Verification items for the finished model (mm, model axes). Face numbers are marked on the shaded views. A direction names the side the tool comes from. Coordinates: 2 decimals unless noted, no trailing zeros. Write each loop counter-clockwise with the first axis right and the second up, starting at its lowest first coordinate (ties: lowest second). Pieces come first, ordered by that corner, then holes. Notation, with made-up numbers: M 84,82 L 116,82 A20 cw 116,103 Z; hole C 82,36 d1. An arc over 180 degrees is marked long. One line per item, written item: value.
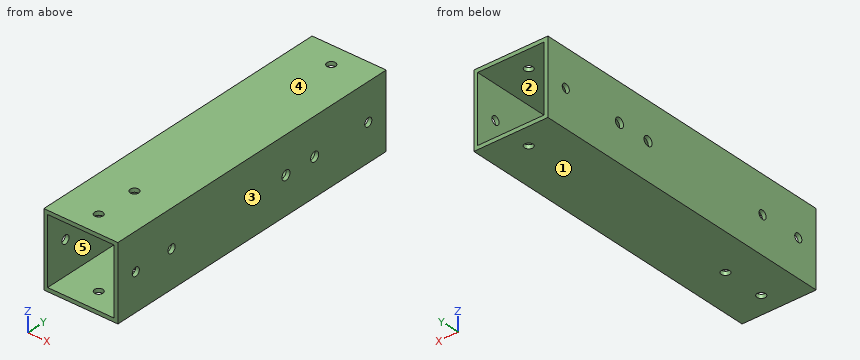
```python
from build123d import *

# Parameters (mm, degrees)
SKETCH1_W           = 35
SKETCH1_H           = 35
SKETCH1_W_2         = 31.4
SKETCH1_H_2         = 31.4
BOSS_EXTRUDE1_DEPTH = 150
SKETCH3_R           = 2
CUT_EXTRUDE1_DEPTH  = 156.020159979
SKETCH4_R           = 2
CUT_EXTRUDE2_DEPTH  = 156.020159979
SKETCH7_R           = 2
CUT_EXTRUDE5_DEPTH  = 40
SKETCH9_R           = 2
CUT_EXTRUDE6_DEPTH  = 40
SKETCH11_R          = 2.25
CUT_EXTRUDE8_DEPTH  = 156.020159979


with BuildPart() as part:
    # Sketch1 → Boss-Extrude1 (new body)
    with BuildSketch(Plane(origin=(0, 0, 0), x_dir=(1, 0, 0), z_dir=(0, 1, 0))):
        Rectangle(SKETCH1_W, SKETCH1_H)
        Rectangle(SKETCH1_W_2, SKETCH1_H_2, mode=Mode.SUBTRACT)
    extrude(amount=BOSS_EXTRUDE1_DEPTH)

    # Sketch3 → Cut-Extrude1 (cut, through all)
    with BuildSketch(Plane.XY.offset(17.5)):
        with Locations((0, 10)):
            Circle(SKETCH3_R)
        with Locations((0, 30)):
            Circle(SKETCH3_R)
    extrude(amount=-CUT_EXTRUDE1_DEPTH, mode=Mode.SUBTRACT)

    # Sketch4 → Cut-Extrude2 (cut, through all)
    with BuildSketch(Plane(origin=(17.5, 0, 0), x_dir=(0, 0, -1), z_dir=(1, 0, 0))):
        with Locations((0, 10)):
            Circle(SKETCH4_R)
        with Locations((0, 30)):
            Circle(SKETCH4_R)
    extrude(amount=-CUT_EXTRUDE2_DEPTH, mode=Mode.SUBTRACT)

    # Sketch7 → Cut-Extrude5 (cut)
    with BuildSketch(Plane(origin=(17.5, 0, 0), x_dir=(0, 0, -1), z_dir=(1, 0, 0))):
        with Locations((0, 140)):
            Circle(SKETCH7_R)
    extrude(amount=-CUT_EXTRUDE5_DEPTH, mode=Mode.SUBTRACT)

    # Sketch9 → Cut-Extrude6 (cut)
    with BuildSketch(Plane.XY.offset(17.5)):
        with Locations((0, 140)):
            Circle(SKETCH9_R)
    extrude(amount=-CUT_EXTRUDE6_DEPTH, mode=Mode.SUBTRACT)

    # Sketch11 → Cut-Extrude8 (cut, through all)
    with BuildSketch(Plane(origin=(17.5, 0, 0), x_dir=(0, 0, -1), z_dir=(1, 0, 0))):
        with Locations((0, 110)):
            Circle(SKETCH11_R)
        with Locations((0, 94)):
            Circle(SKETCH11_R)
    extrude(amount=-CUT_EXTRUDE8_DEPTH, mode=Mode.SUBTRACT)


solid = part.part
```
Item 1: Draft check along X on the marked faces 1, 2 and 3. Enter one of: released by +X, released by -X, zero draft, split by the parting line, or undercut.
The answers:
face 1: zero draft
face 2: undercut
face 3: released by +X
Item 2: Cross-section at D-D, the plane x = 0. Give the number of separate pieces and of enclosed holes in the cut face, and give its area (3 significant figures).
The answers:
separate pieces: 8
enclosed holes: 0
area: 497 mm²
Item 3: Cross-section at A-A, the plane y = 30. Enter the section's corners in (x, z).
The answers:
outline: M -17.5,-17.5 L -2,-17.5 L -2,-15.7 L -15.7,-15.7 L -15.7,-2 L -17.5,-2 Z; M -17.5,2 L -15.7,2 L -15.7,15.7 L -2,15.7 L -2,17.5 L -17.5,17.5 Z; M 2,-17.5 L 17.5,-17.5 L 17.5,-2 L 15.7,-2 L 15.7,-15.7 L 2,-15.7 Z; M 2,15.7 L 15.7,15.7 L 15.7,2 L 17.5,2 L 17.5,17.5 L 2,17.5 Z
Item 4: Cross-section at C-C, the plane y = 110. Enter the section's corners in (x, z).
The answers:
outline: M -17.5,-17.5 L 17.5,-17.5 L 17.5,-2.25 L 15.7,-2.25 L 15.7,-15.7 L -15.7,-15.7 L -15.7,-2.25 L -17.5,-2.25 Z; M -17.5,2.25 L -15.7,2.25 L -15.7,15.7 L 15.7,15.7 L 15.7,2.25 L 17.5,2.25 L 17.5,17.5 L -17.5,17.5 Z
Item 5: Scan lines: line 1 (Y direction, x = -16, z = 0); line 2 (Y direction, x = 0, z = -16.35); line 3 (X direction, y = 137, z = -0.5). Record each from-to range of solid material in increasing order.
The answers:
line 1: y = 0 to 8, 12 to 28, 32 to 91.75, 96.25 to 107.75, 112.25 to 138, 142 to 150
line 2: y = 0 to 8, 12 to 28, 32 to 138, 142 to 150
line 3: x = -17.5 to -15.7, 15.7 to 17.5
Item 6: Cross-section at B-B, the plane z = 14. Enter the section's corners in (x, y).
The answers:
outline: M -17.5,0 L -15.7,0 L -15.7,150 L -17.5,150 Z; M 15.7,0 L 17.5,0 L 17.5,150 L 15.7,150 Z
Item 7: Access from +Z, -Z, +X, -X, +Y, -Y to the whole of each face (thin tool, end or side, straight path). Record for the marked faces 4 and 5.
The answers:
face 4: +Z, +X, -X, +Y, -Y
face 5: +Y, -Y
